```python
from build123d import *

# Parameters (mm, degrees)
F0_R     = 38.1
F0_R_2   = 4.445
F0_R_3   = 23.1824441608
F1_DEPTH = 50.8
F0_R_4   = 8.0064033383
F2_DEPTH = 63.5
F3_DEPTH = 68.58
F4_DEPTH = 2.54
F5_DEPTH = 25.4
F6_DEPTH = 38.1


# Not quite as in the source:
# - a fillet or chamfer that OpenCascade refuses, or shapes differently, is made with other operations: its cross-section is extruded or revolved along the edge and cut away or added


with BuildPart() as f1:
    # F0 (on Top) → F1 (new body)
    with BuildSketch(Plane.XY):
        Circle(F0_R)
        with Locations((-21.3879767226, -21.3879767226)):
            Circle(F0_R_2, mode=Mode.SUBTRACT)
        with Locations((0, -30.2471667528)):
            Circle(F0_R_2, mode=Mode.SUBTRACT)
        with Locations((21.3879767226, -21.3879767226)):
            Circle(F0_R_2, mode=Mode.SUBTRACT)
        with Locations((-30.2471667528, 0)):
            Circle(F0_R_2, mode=Mode.SUBTRACT)
        with Locations((-21.3879767226, 21.3879767226)):
            Circle(F0_R_2, mode=Mode.SUBTRACT)
        Circle(F0_R_3, mode=Mode.SUBTRACT)
        with Locations((30.2471667528, 0)):
            Circle(F0_R_2, mode=Mode.SUBTRACT)
        with Locations((0, 30.2471667528)):
            Circle(F0_R_2, mode=Mode.SUBTRACT)
        with Locations((21.3879767226, 21.3879767226)):
            Circle(F0_R_2, mode=Mode.SUBTRACT)
    extrude(amount=F1_DEPTH)

    # F0 (on Top) → F2 (join)
    with BuildSketch(Plane.XY):
        Circle(F0_R_3)
        with Locations((-8.6240968668, -12.7810694279)):
            Circle(F0_R_2, mode=Mode.SUBTRACT)
        with Locations((9.4905268716, -12.1515711819)):
            Circle(F0_R_2, mode=Mode.SUBTRACT)
        with Locations((-14.8205118576, 4.2524358628)):
            Circle(F0_R_2, mode=Mode.SUBTRACT)
        with Locations((-0.5354831918, 15.4092193261)):
            Circle(F0_R_2, mode=Mode.SUBTRACT)
        Circle(F0_R_4, mode=Mode.SUBTRACT)
        with Locations((14.4895650446, 5.2709854208)):
            Circle(F0_R_2, mode=Mode.SUBTRACT)
    extrude(amount=F2_DEPTH)

    # F0 (on Top) → F3 (join)
    with BuildSketch(Plane.XY):
        Circle(F0_R_4)
        Circle(F0_R_2, mode=Mode.SUBTRACT)
    extrude(amount=F3_DEPTH)

    # F0 (on Top) → F4 (join)
    with BuildSketch(Plane.XY):
        with Locations((-30.2471667528, 0)):
            Circle(F0_R_2)
        with Locations((-21.3879767226, -21.3879767226)):
            Circle(F0_R_2)
        with Locations((0, -30.2471667528)):
            Circle(F0_R_2)
        with Locations((21.3879767226, -21.3879767226)):
            Circle(F0_R_2)
        with Locations((21.3879767226, 21.3879767226)):
            Circle(F0_R_2)
        with Locations((0, 30.2471667528)):
            Circle(F0_R_2)
        with Locations((-21.3879767226, 21.3879767226)):
            Circle(F0_R_2)
        with Locations((30.2471667528, 0)):
            Circle(F0_R_2)
    extrude(amount=F4_DEPTH)

    # F0 (on Top) → F5 (join)
    with BuildSketch(Plane.XY):
        with Locations((-8.6240968668, -12.7810694279)):
            Circle(F0_R_2)
        with Locations((9.4905268716, -12.1515711819)):
            Circle(F0_R_2)
        with Locations((14.4895650446, 5.2709854208)):
            Circle(F0_R_2)
        with Locations((-0.5354831918, 15.4092193261)):
            Circle(F0_R_2)
        with Locations((-14.8205118576, 4.2524358628)):
            Circle(F0_R_2)
    extrude(amount=F5_DEPTH)

    # F0 (on Top) → F6 (join)
    with BuildSketch(Plane.XY):
        Circle(F0_R_2)
    extrude(amount=F6_DEPTH)

    # F7: chamfer of 5.08 on 3 edges, made by hand

    # F7_s1 → F7_t2 (revolve, cut)
    with BuildSketch(Plane.XZ):
        Polygon((38.1, 45.72), (33.02, 50.8), (38.1, 50.8), align=None)
    revolve(axis=Axis((0, 0, 50.8), (0, 0, 1)), mode=Mode.SUBTRACT)

    # F7_s3 → F7_t4 (revolve, cut)
    with BuildSketch(Plane.XZ):
        Polygon((23.1824441608, 58.42), (18.1024441608, 63.5), (23.1824441608, 63.5), align=None)
    revolve(axis=Axis((0, 0, 63.5), (0, 0, 1)), mode=Mode.SUBTRACT)


with BuildPart() as f7_tool6:
    # F7_s7 → F7_t8 (revolve)
    with BuildSketch(Plane.XZ):
        Polygon((8.0064033383, 63.5), (2.9264033383, 68.58), (8.0064033383, 68.58), align=None)
    revolve(axis=Axis((0, 0, 68.58), (0, 0, 1)))

    split(bisect_by=Plane.XY.offset(63.5), keep=Keep.TOP)


with BuildPart() as f1_1:
    add(f1.part)

    # F7_t5: cut F7_tool6
    add(f7_tool6.part, mode=Mode.SUBTRACT)


solid = f1_1.part
```
Source: CAD feature listing. Evaluate the final solid. Frame: model axes, mm. Give positions to 0.01 mm unless a question says otherwise; leave off trailing zeros. Write each loop counter-clockwise with the first axis right and the second up, starting at its lowest first coordinate (ties: lowest second). Pieces come first, ordered by that corner, then holes.
1. Section query A-A (z = 59.5). Return the cut outline in (x, y) (3 decimals).
2. Material intervals for line 1 along Y through (x, z) = (0, 21); line 2 along X through (y, z) = (4, 49); line 3 along Y through (x, z) = (-17.5, 24.5), sorted ascending.
3. Section query B-B (z = 22). Count the separate pieces of the cut face and the enclosed holes in it, then the cut area to 3 significant figures.
4. First-contact query: pin 1 (8 mm diameter, centred on x = 9.49, y = -12.15, fed in from +Z); pin 2 (3 mm diameter, centred on y = 1, z = 10, fed in from -X); pin 3 (8 mm diameter, centred on y = 29.5, z = 48, fed in from -X); pin 4 (5 mm diameter, centred on x = -16.5, z = 58, fed in from +Y). Flat tips, straight axial feed; report the tip coordinate or a pass-through.
5. Pull-direction query (Y, two-part tool) for faces 1 (the face through (-10, 22, 50.8)), 2 (the face through (21, 21, 2.54)), 3 (the face through (10.697, -20.567, 54.557)); classes: +Y half, -Y half, draft (parallel to the pull), parting line (faces both ways), or undercut.
6. Section query C-C (x = 0). Return the cut outline in (y, z) (3 decimals), then the cut area to 3 significant figures.
Output values:
1. outline: circle Ø44.205 at (0, 0); hole circle Ø8.89 at (-14.821, 4.252); hole circle Ø8.89 at (-8.624, -12.781); hole circle Ø8.89 at (-0.535, 15.409); hole circle Ø8.89 at (0, 0); hole circle Ø8.89 at (9.491, -12.152); hole circle Ø8.89 at (14.49, 5.271)
2. line 1: y = -38.1 to -34.69, -25.8 to 25.8, 34.69 to 38.1
2. line 2: x = -34.59 to -32.19, -28.31 to -19.26, -10.38 to -1.94, 1.94 to 10.23, 18.75 to 28.31, 32.19 to 34.59
2. line 3: y = -33.84 to -23.54, -19.23 to 19.23, 23.54 to 33.84
3. separate pieces: 1
3. enclosed holes: 8
3. area: 4,060 mm2
4. pin 1: stops at z = 25.4
4. pin 2: stops at x = -38.1
4. pin 3: stops at x = -27.65
4. pin 4: stops at y = 18.48
5. face 1: draft
5. face 2: undercut
5. face 3: parting line
6. outline: (-38.1, 0) - (38.1, 0) - (38.1, 45.72) - (34.692, 49.128) - (34.692, 2.54) - (25.802, 2.54) - (25.802, 50.8) - (23.182, 50.8) - (23.182, 58.42) - (19.822, 61.781) - (19.822, 25.4) - (10.997, 25.4) - (10.997, 63.5) - (8.006, 63.5) - (4.445, 67.061) - (4.445, 38.1) - (-4.445, 38.1) - (-4.445, 67.061) - (-8.006, 63.5) - (-18.102, 63.5) - (-23.182, 58.42) - (-23.182, 50.8) - (-25.802, 50.8) - (-25.802, 2.54) - (-34.692, 2.54) - (-34.692, 49.128) - (-38.1, 45.72) - close
6. area: 3,010 mm2
